The model under review builds one solid part; all positions refer to its coordinate system, in mm. Face numbers are marked on the shaded views. A direction names the side the tool comes from. Give positions to 0.01 mm unless a question says otherwise; leave off trailing zeros. Loops run counter-clockwise (first coordinate to the right, second up) from the corner with the lowest first, then second, coordinate; pieces in that order, holes last. Notation, with made-up numbers: (57.5, 5.5) - (109.5, 5.5) arc R19 ccw to (109.5, 35.5) - close; hole circle Ø2 at (-26.75, 76). An arc over 180 degrees is marked (long way). Return JSON: item names as keys, results as strings. Group by question number.
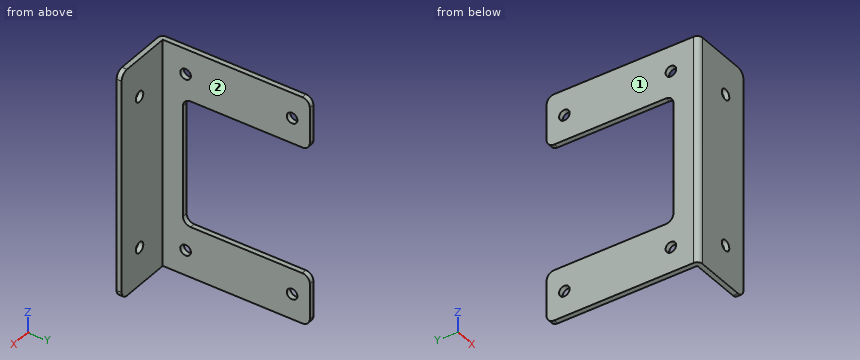
```python
from build123d import *

# Parameters (mm, degrees)
EXTRUDE_1_DEPTH     = 45
SKETCH_2_R          = 2.1
SKETCH_2_W          = 50
SKETCH_2_H          = 50
CUT_EXTRUDE_2_DEPTH = 113.055777281
SKETCH_3_R          = 2.1
CUT_EXTRUDE_3_DEPTH = 113.055777281
FILLET_1_R          = 3


with BuildPart() as part:
    # ｽｹｯﾁ1 → ﾎﾞｽ - 押し出し1 (new, symmetric)
    with BuildSketch(Plane.XY):
        with BuildLine():
            Line((0, -39.531388125), (2, -39.531388125))
            Line((2, -39.531388125), (2, -97.531388125))
            Line((2, -97.531388125), (25, -97.531388125))
            Line((25, -97.531388125), (25, -99.531388125))
            Line((25, -99.531388125), (2, -99.531388125))
            ThreePointArc((2, -99.531388125), (0.585786438, -98.945601688), (0, -97.531388125))
            Line((0, -97.531388125), (0, -39.531388125))
        make_face()
    extrude(amount=EXTRUDE_1_DEPTH, both=True)

    # ｽｹｯﾁ2 → ｶｯﾄ - 押し出し2 (cut, through all)
    with BuildSketch(Plane(origin=(0, 0, 0), x_dir=(0, 0, -1), z_dir=(1, 0, 0))):
        with Locations(Location((-35, -46.531388125, 0), (0, 0, 270))):
            Circle(SKETCH_2_R)
        with Locations(Location((-35, -88.531388125, 0), (0, 0, 270))):
            Circle(SKETCH_2_R)
        with Locations(Location((35, -88.531388125, 0), (0, 0, 180))):
            Circle(SKETCH_2_R)
        with Locations(Location((35, -46.531388125, 0), (0, 0, 180))):
            Circle(SKETCH_2_R)
        with Locations((0, -64.531388125)):
            Rectangle(SKETCH_2_W, SKETCH_2_H)
    extrude(amount=CUT_EXTRUDE_2_DEPTH, mode=Mode.SUBTRACT)

    # ｽｹｯﾁ3 → ｶｯﾄ - 押し出し3 (cut, through all)
    with BuildSketch(Plane(origin=(0, 0, 0), x_dir=(1, 0, 0), z_dir=(0, 1, 0))):
        with Locations(Location((15, 30, 0), (0, 0, 270))):
            Circle(SKETCH_3_R)
        with Locations(Location((15, -30, 0), (0, 0, 270))):
            Circle(SKETCH_3_R)
    extrude(amount=-CUT_EXTRUDE_3_DEPTH, mode=Mode.SUBTRACT)

    # ﾌｨﾚｯﾄ1
    fillet_1_edges = [part.edges().sort_by_distance(p)[0] for p in [
        (25, -98.531388125, 45),
        (1, -39.531388125, -25),
        (1, -39.531388125, 45),
        (1, -39.531388125, 25),
        (1, -89.531388125, 25),
        (1, -89.531388125, -25),
        (1, -39.531388125, -45),
        (25, -98.531388125, -45),
    ]]
    fillet(fillet_1_edges, radius=FILLET_1_R)


solid = part.part
```
1) We need section C-C, the plane z = 29. Write out the cut boundary in (x, y), plus the area to 3 significant figures.
2) Tool access review of the marked faces 1 and 2: name each direction out of +Z, -Z, +X, -X, +Y, -Y from which nothing blocks a thin tool from reaching the whole face with its end or side.
3) We need section A-A, the plane z = -35. Write out the cut boundary in (x, y), plus the area to 3 significant figures.
4) For pin 1 Ø1 at (x, z) = (1.5, -6.5) entering from +Y; pin 2 Ø5.5 at (x, z) = (15, -30) entering from +Y; pin 3 Ø6.5 at (y, z) = (-88.53, -35) entering from +X, all flat-tipped, find the tip position at first contact; note any pin that passes through.
5) We need section B-B, the plane y = -61. Write out the cut boundary in (x, z), plus the area to 3 significant figures.
6) To check wall thickness, follow line 1 (Y direction, x = 1.4, z = -35); line 2 (Y direction, x = 8, z = 14.5); line 3 (X direction, y = -93.5, z = 28.5). State the ranges of each line that lie inside material, in increasing order.
7) We need section D-D, the plane z = -15. Write out the cut boundary in (x, y), plus the area to 3 significant figures.
Findings:
{
 "1": {"outline": "(0, -97.53) arc R2 ccw to (2, -99.53) - (13.15, -99.53) - (13.15, -97.53) - (2, -97.53) - (2, -39.53) - (0, -39.53) - close; (16.85, -99.53) - (25, -99.53) - (25, -97.53) - (16.85, -97.53) - close", "area": "158 mm^2"},
 "2": {"face 1": "+Z, -Z, -X, +Y, -Y", "face 2": "+Z, -Z, +X, +Y"},
 "3": {"outline": "(0, -97.53) arc R2 ccw to (2, -99.53) - (25, -99.53) - (25, -97.53) - (2, -97.53) - (2, -90.63) - (0, -90.63) - close; (0, -86.43) - (2, -86.43) - (2, -48.63) - (0, -48.63) - close; (0, -44.43) - (2, -44.43) - (2, -39.53) - (0, -39.53) - close", "area": "148 mm^2"},
 "4": {"pin 1": "stops at y = -89.53", "pin 2": "stops at y = -97.53", "pin 3": "stops at x = 2"},
 "5": {"outline": "(0, -45) - (2, -45) - (2, -25) - (0, -25) - close; (0, 25) - (2, 25) - (2, 45) - (0, 45) - close", "area": "80.0 mm^2"},
 "6": {"line 1": "y = -99.44 to -90.63, -86.43 to -48.63, -44.43 to -39.53", "line 2": "y = -99.53 to -97.53", "line 3": "x = 0 to 2"},
 "7": {"outline": "(0, -97.53) arc R2 ccw to (2, -99.53) - (25, -99.53) - (25, -97.53) - (2, -97.53) - (2, -89.53) - (0, -89.53) - close", "area": "65.1 mm^2"}
}
